Geometry check sheet. Reference: drawing and pictorial views, mm from the part's lowest x, y, z. A direction names the side the tool comes from. Coordinates: 2 decimals unless noted, no trailing zeros. Order: outer loops, then holes, each group sorted by start corner. A loop starts at its lowest first (then second) coordinate and runs counter-clockwise, first axis right, second up. Notation, with made-up numbers: M 12.25,-3.75 L 16.25,-3.75 A22 ccw 16.25,19.25 Z; hole C 65,48.25 d1. An arc over 180 degrees is marked long. Return JSON: item names as keys, results as strings.
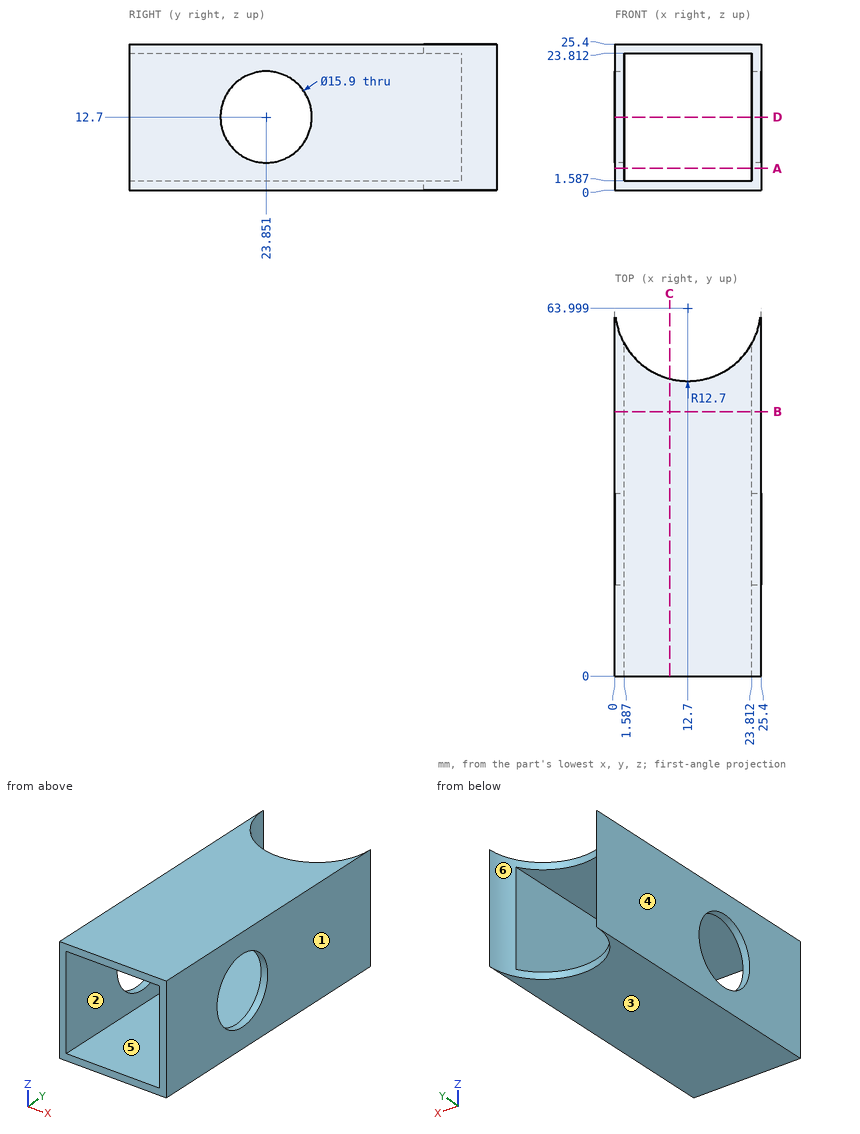
Q1. Tool access check on the marked faces 1 and 2. Record the directions out of +Z, -Z, +X, -X, +Y, -Y that give a thin tool (end or side, any length) a straight path to the whole face; none if there is none.
Values:
{"face 1": "+Z, -Z, +X, +Y, -Y", "face 2": "+Y, -Y"}
Q2. Cross-section at D-D, the plane z = 12.7. Record the boundary of the cut face in (x, y).
Values:
{"outline": "M 0,0 L 1.59,0 L 1.59,15.9 L 0,15.9 Z; M 0,31.8 L 1.59,31.8 L 1.59,57.85 A12.7 cw 0,64 Z; M 23.81,0 L 25.4,0 L 25.4,15.9 L 23.81,15.9 Z; M 23.81,31.8 L 25.4,31.8 L 25.4,64 A12.7 cw 23.81,57.85 Z"}
Q3. Draft check along X on the marked faces 3, 4, 5 and 6. Enter one of: pulls with the +X half, pulls with the -X half, needs draft (parallel to the pull), parting line crosses it, or undercut.
Values:
{"face 3": "needs draft", "face 4": "pulls with the -X half", "face 5": "undercut", "face 6": "undercut"}
Q4. Cross-section at A-A, the plane z = 3.75. Record the boundary of the cut face in (x, y), and give its area (3 significant figures).
Values:
{"outline": "M 0,0 L 1.59,0 L 1.59,57.85 A12.7 cw 0,64 Z; M 23.81,0 L 25.4,0 L 25.4,64 A12.7 cw 23.81,57.85 Z", "area": "190 mm^2"}
Q5. Cross-section at C-C, the plane x = 9.5. Record the boundary of the cut face in (y, z), and give its area (3 significant figures).
Values:
{"outline": "M 0,0 L 51.71,0 L 51.71,1.59 L 0,1.59 Z; M 0,23.81 L 51.71,23.81 L 51.71,25.4 L 0,25.4 Z", "area": "164 mm^2"}
Q6. Cross-section at B-B, the plane y = 46. Record the boundary of the cut face in (x, z).
Values:
{"outline": "M 0,0 L 25.4,0 L 25.4,25.4 L 0,25.4 Z; hole M 1.59,1.59 L 23.81,1.59 L 23.81,23.81 L 1.59,23.81 Z"}
Q7. Material ranges on line 1 along Z through (x, y) = (18, 28); line 2 along Y through (x, z) = (24.25, 12.7) (1 decimal), recorded low to high.
Values:
{"line 1": "0 to 1.59, 23.81 to 25.4", "line 2": "0 to 15.9, 31.8 to 58.7"}
